Autodesk Inventor part; units mm, degrees
ref_plane "Work Plane3" through (-15.6216, -29.5135, 0) normal (0, -1, 0) x (1, 0, 0)
ref_plane "Work Plane4" through (12.3784, -29.5135, -28) normal (0, 0, -1) x (-1, 0, 0)
ref_plane "Work Plane5" through (-15.6216, -1.5135, 30) normal (0, 1, 0) x (1, 0, 0)
sketch "Sketch1" plane through (0, 0, 0) normal (0, 0, 1) x (1, 0, 0)
  line L0 (-11.6216, -5.5135) -> (8.3784, -5.5135)
  line L1 (8.3784, -5.5135) -> (8.3784, -25.5135)
  line L2 (8.3784, -25.5135) -> (-11.6216, -25.5135)
  line L3 (-11.6216, -25.5135) -> (-11.6216, -5.5135)
  line L4 (-15.6216, -1.5135) -> (12.3784, -1.5135)
  line L5 (12.3784, -1.5135) -> (12.3784, -29.5135)
  line L6 (12.3784, -29.5135) -> (-15.6216, -29.5135)
  line L7 (-15.6216, -29.5135) -> (-15.6216, -1.5135)
  point P0 (0, 0)
  dimension "d0" = 20
  dimension "d1" = 20
  dimension "d2" = 4
  dimension "d3" = 4
  dimension "d4" = 4
  dimension "d5" = 4
extrude "Extrusion1" add sketch "Sketch1" along normal blind 30
ref_plane "Work Plane3" through (-15.6216, -29.5135, 0) normal (0, -1, 0) x (1, 0, 0)
sketch "Sketch2" plane through (-15.6216, -29.5135, 0) normal (0, -1, 0) x (1, 0, 0)
  line L0 (0, 0) -> (28, 0)
  line L1 (28, 0) -> (28, -28)
  line L2 (28, -28) -> (0, -28)
  line L3 (0, -28) -> (0, 0)
  line L4 (24, -24) -> (4, -24)
  line L5 (4, -24) -> (4, -4)
  line L6 (4, -4) -> (24, -4)
  line L7 (24, -4) -> (24, -24)
  point P0 (15.6216, 0)
  point P1 (0, -14)
  dimension "d10" = 28
  dimension "d11" = 28
  dimension "d12" = 4
  dimension "d13" = 4
  dimension "d14" = 4
  dimension "d15" = 4
extrude "Extrusion2" add sketch "Sketch2" against normal blind 50
ref_plane "Work Plane4" through (12.3784, -29.5135, -28) normal (0, 0, -1) x (-1, 0, 0)
sketch "Sketch3" plane through (12.3784, -29.5135, -28) normal (0, 0, -1) x (-1, 0, 0)
  circle A0 centre (14, 35) radius 2.5
  circle A1 centre (14, 15) radius 2.5
  line L0 (28, 0) -> (28, 50)
  line L1 (28, 0) -> (0, 0)
  point P0 (12.3784, 29.5135)
  dimension "d19" = 14
  dimension "d20" = 14
  dimension "d21" = 20
  dimension "d22" = 15
  dimension "d23" = 5
  dimension "d24" = 5
ref_plane "Work Plane5" through (-15.6216, -1.5135, 30) normal (0, 1, 0) x (1, 0, 0)
sketch "Sketch4" plane through (-15.6216, -1.5135, 30) normal (0, 1, 0) x (1, 0, 0)
  circle A0 centre (14, 15) radius 2.5
  line L0 (28, 30) -> (28, 0)
  line L1 (28, 0) -> (0, 0)
  point P0 (15.6216, 30)
  dimension "d26" = 5
  dimension "d27" = 14
  dimension "d28" = 15
ref_plane "Work Plane6" through (-15.6216, -29.5135, 30) normal (0, -1, 0) x (1, 0, 0)
sketch "Sketch5" plane through (-15.6216, -29.5135, 30) normal (0, -1, 0) x (1, 0, 0)
  circle A0 centre (14, -15) radius 2.5
  line L0 (0, -30) -> (0, 0)
  line L1 (24, 0) -> (4, 0)
  point P0 (15.6216, -30)
  dimension "d30" = 5
  dimension "d31" = 14
  dimension "d32" = 15
extrude "Extrusion3" cut sketch "Sketch4" against normal blind 4
extrude "Extrusion4" cut sketch "Sketch5" against normal blind 4
extrude "Extrusion5" cut sketch "Sketch3" against normal blind 4
fillet "Fillet1" radius 2 8 edges at (12.3784, -1.5135, 15) (12.3784, 9.4865, 0) (12.3784, -29.5135, 1) (12.3784, -4.5135, -28) (-15.6216, 9.4865, 0) (-15.6216, -1.5135, 15) (-15.6216, -4.5135, -28) (-15.6216, -29.5135, 1)
fillet "Fillet2" radius 0.5 31 edges at (-1.6216, -29.5135, -24) (8.3784, -29.5135, -14) (-11.6216, -29.5135, -14) (-1.6216, -29.5135, -4) (11.7926, -28.9277, -27.4142) (-15.0358, -28.9277, -27.4142) (-1.6216, -29.5135, -28) (-1.6216, 20.4865, -24) (-11.6216, 20.4865, -14) (8.3784, 20.4865, -14) (-1.6216, 20.4865, -4) (-15.0358, 20.4865, -27.4142) (-15.6216, 20.4865, -14) (-15.0358, 20.4865, -0.5858) (-1.6216, 20.4865, 0) (11.7926, 20.4865, -0.5858) (12.3784, 20.4865, -14) (11.7926, 20.4865, -27.4142) (-1.6216, 20.4865, -28) (-1.6216, -25.5135, 30) (8.3784, -15.5135, 30) (-1.6216, -5.5135, 30) (-11.6216, -15.5135, 30) (11.7926, -28.9277, 30) (12.3784, -15.5135, 30) (11.7926, -2.0993, 30) (-1.6216, -1.5135, 30) (-15.0358, -2.0993, 30) (-15.6216, -15.5135, 30) (-15.0358, -28.9277, 30) (-1.6216, -29.5135, 30)
ref_plane "Work Plane7" through (-13.6216, -29.5135, 29.5) normal (0, -1, 0) x (1, 0, 0)
sketch "Sketch6" plane through (-13.6216, -29.5135, 29.5) normal (0, -1, 0) x (1, 0, 0)
  line L0 (23.2157, -54.9948) -> (0.8161, -54.9948)
  line L1 (0.8161, -54.9948) -> (0.8161, -31.6008)
  line L2 (0.8161, -31.6008) -> (23.2157, -31.6008)
  line L3 (23.2157, -31.6008) -> (23.2157, -54.9948)
  point P0 (13.6216, -29.5)
extrude "Extrusion6" add sketch "Sketch6" against normal blind 4
properties part number "fixed_joint"
The listing builds one solid part. Answer for the finished solid, in the listing's coordinates (mm). A direction names the side the tool comes from. Round coordinates to 2 decimals unless told otherwise and drop trailing zeros. Loops run counter-clockwise (first coordinate to the right, second up) from the corner with the lowest first, then second, coordinate; pieces in that order, holes last.
1) A cutting plane is placed at D-D on z = -9. Determine the outline of the cut face in (x, y), plus the area to 3 significant figures.
Outcome:
outline: (-15.62, -27.51) arc R2 ccw to (-13.62, -29.51) - (10.38, -29.51) arc R2 ccw to (12.38, -27.51) - (12.38, 19.99) arc R0.5 ccw to (11.88, 20.49) - (8.88, 20.49) arc R0.5 ccw to (8.38, 19.99) - (8.38, -25.51) - (-11.62, -25.51) - (-11.62, 19.99) arc R0.5 ccw to (-12.12, 20.49) - (-15.12, 20.49) arc R0.5 ccw to (-15.62, 19.99) - close
area: 478 mm2
2) For faces 1 (the face through (-11.622, -3, -14)), 2 (the face through (-15.05, 8.4, -0.6)), 3 (the face through (-11.622, -16, 15)), 4 (the face through (-2, 9, 0)), determine the directions among +Z, -Z, +X, -X, +Y, -Y from which every point of the face is accessible in a straight line to the end or side of a thin tool.
Outcome:
face 1: +Y
face 2: +Z, -X, +Y
face 3: +Z
face 4: +Z, +X, -X, +Y
3) A cutting plane is placed at B-B on z = 15. Determine the outline of the cut face in (x, y).
Outcome:
outline: (-15.62, -27.51) arc R2 ccw to (-13.62, -29.51) - (-4.12, -29.51) - (-4.12, -25.51) - (-11.62, -25.51) - (-11.62, -5.51) - (-4.12, -5.51) - (-4.12, -1.51) - (-13.62, -1.51) arc R2 ccw to (-15.62, -3.51) - close; (0.88, -29.51) - (10.38, -29.51) arc R2 ccw to (12.38, -27.51) - (12.38, -3.51) arc R2 ccw to (10.38, -1.51) - (0.88, -1.51) - (0.88, -5.51) - (8.38, -5.51) - (8.38, -25.51) - (0.88, -25.51) - close
4) A cutting plane is placed at C-C on x = 2. Determine the outline of the cut face in (y, z).
Outcome:
outline: (-29.51, -27.5) arc R0.5 ccw to (-29.01, -28) - (19.99, -28) arc R0.5 ccw to (20.49, -27.5) - (20.49, -24.5) arc R0.5 ccw to (19.99, -24) - (-25.51, -24) - (-25.51, -4) - (19.99, -4) arc R0.5 ccw to (20.49, -3.5) - (20.49, -0.5) arc R0.5 ccw to (19.99, 0) - (-1.51, 0) - (-1.51, 29.5) arc R0.5 ccw to (-2.01, 30) - (-5.01, 30) arc R0.5 ccw to (-5.51, 29.5) - (-5.51, 0) - (-25.51, 0) - (-25.51, 29.5) arc R0.5 ccw to (-26.01, 30) - (-29.01, 30) arc R0.5 ccw to (-29.51, 29.5) - close
5) A cutting plane is placed at A-A on y = -24. Determine the outline of the cut face in (x, z).
Outcome:
outline: (-15.62, -26) arc R2 ccw to (-13.62, -28) - (10.38, -28) arc R2 ccw to (12.38, -26) - (12.38, 29.5) arc R0.5 ccw to (11.88, 30) - (8.88, 30) arc R0.5 ccw to (8.38, 29.5) - (8.38, 0) - (-11.62, 0) - (-11.62, 29.5) arc R0.5 ccw to (-12.12, 30) - (-15.12, 30) arc R0.5 ccw to (-15.62, 29.5) - close; hole (-11.62, -24) - (8.38, -24) - (8.38, -4) - (-11.62, -4) - close
6) For a pull along Z with two mould halves and no side action, classify faces 5 (the face through (-2, -3, -4)), 6 (the face through (-15.622, -9, -5)), 7 (the face through (-15.02, -4.17, -27.43)) as released by +Z, released by -Z, zero draft, split by the parting line, or undercut.
Outcome:
face 5: undercut
face 6: zero draft
face 7: released by -Z
7) Consider line 1 (X direction, y = 11.5, z = -17); line 2 (Z direction, x = -9, y = 6.5); line 3 (Y direction, x = -7, z = 27). Determine where each line is inside the solid, lowest interval first.
Outcome:
line 1: x = -15.62 to -11.62, 8.38 to 12.38
line 2: z = -28 to -24, -4 to 0
line 3: y = -29.51 to -25.51, -5.51 to -1.51
8) Given P1, Ø3, axis at x = -1.62, y = -14.51, coming from the +Z side; P2, Ø4, axis at x = 7, y = -20, coming from the +Z side; P3, Ø12, axis at x = -0.5, z = 7, coming from the +Y side; P4, Ø4, axis at x = -5.5, z = -19, coming from the +Y side, each flat-ended and moving along its own axis, determine where each tip first touches the part or whether it passes through.
Outcome:
P1: stops at z = 0
P2: stops at z = 30
P3: stops at y = -1.51
P4: stops at y = -25.51
